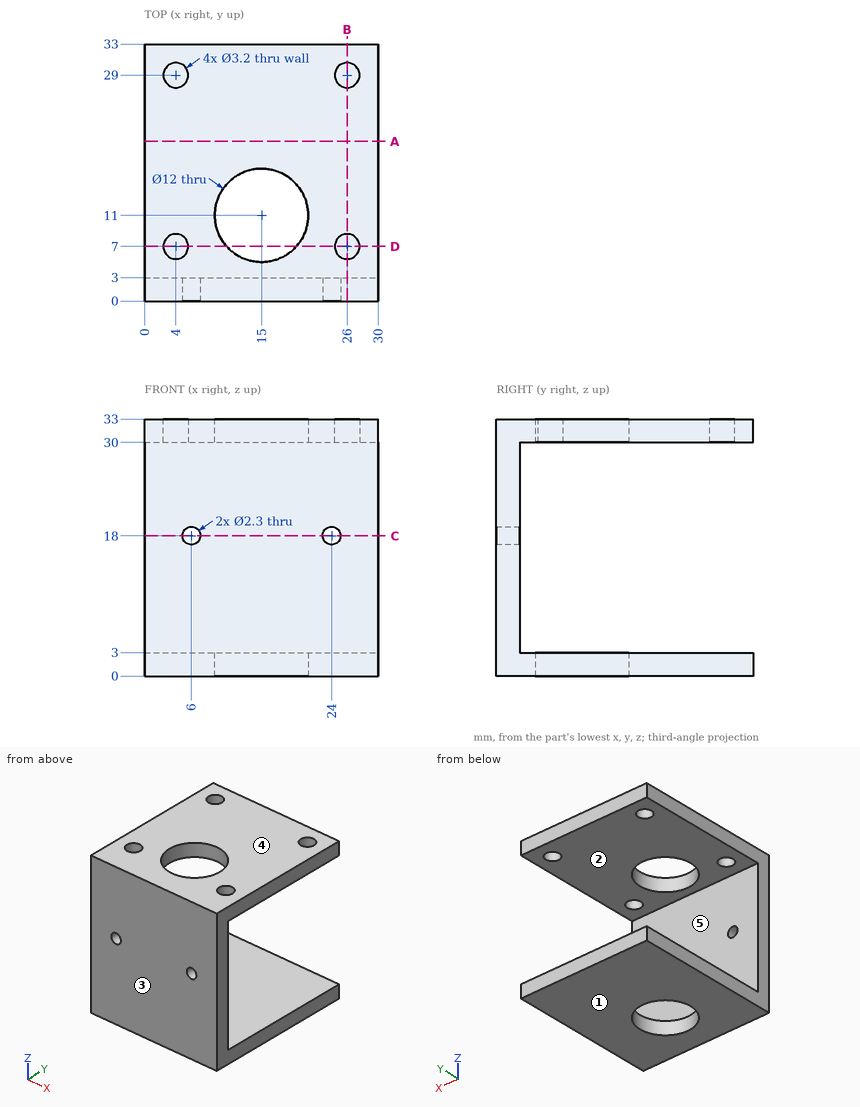
Here's the drawing with two shaded views (mm, measured from the low corner). I have some questions. A direction names the side the tool comes from. Round coordinates to 2 decimals unless told otherwise and drop trailing zeros. Loops run counter-clockwise (first coordinate to the right, second up) from the corner with the lowest first, then second, coordinate; pieces in that order, holes last.
1. Suppose I cut it at D-D, the plane y = 7. Please give me the cut outline in (x, z).
Answers:
outline: (0, 0) - (10.53, 0) - (10.53, 3) - (0, 3) - close; (0, 30) - (2.4, 30) - (2.4, 33) - (0, 33) - close; (5.6, 30) - (10.53, 30) - (10.53, 33) - (5.6, 33) - close; (19.47, 0) - (30, 0) - (30, 3) - (19.47, 3) - close; (19.47, 30) - (24.4, 30) - (24.4, 33) - (19.47, 33) - close; (27.6, 30) - (30, 30) - (30, 33) - (27.6, 33) - close
2. Suppose I cut it at A-A, the plane y = 20.5. Please give me the cut outline in (x, z).
Answers:
outline: (0, 0) - (30, 0) - (30, 3) - (0, 3) - close; (0, 30) - (30, 30) - (30, 33) - (0, 33) - close
3. If I drill on probe 1 along Y at (x, z) = (26, 31.8); probe 2 along X at (y, z) = (1, 18); probe 3 along Z at (x, y) = (24.5, 24), over which ranges is the centre line in solid material (lowest first)?
Answers:
probe 1: y = 0 to 5.4, 8.6 to 27.4, 30.6 to 33
probe 2: x = 0 to 4.85, 7.15 to 22.85, 25.15 to 30
probe 3: z = 0 to 3, 30 to 33
4. Thinking about a two-plate mould opening in Z: for the marked faces 1, 2 and 3, which applies, released by +Z, released by -Z, zero draft, split by the parting line, or undercut?
Answers:
face 1: released by -Z
face 2: undercut
face 3: zero draft
5. Suppose I cut it at B-B, the plane x = 26. Please give me the cut outline in (y, z).
Answers:
outline: (0, 0) - (33, 0) - (33, 3) - (3, 3) - (3, 30) - (5.4, 30) - (5.4, 33) - (0, 33) - close; (8.6, 30) - (27.4, 30) - (27.4, 33) - (8.6, 33) - close; (30.6, 30) - (33, 30) - (33, 33) - (30.6, 33) - close
6. Suppose I cut it at C-C, the plane z = 18. Please give me the cut outline in (x, y).
Answers:
outline: (0, 0) - (4.85, 0) - (4.85, 3) - (0, 3) - close; (7.15, 0) - (22.85, 0) - (22.85, 3) - (7.15, 3) - close; (25.15, 0) - (30, 0) - (30, 3) - (25.15, 3) - close
7. Will these pins go through, and if not, where does the flat tip stop? pin 1 (12 mm diameter, centred on y = 13.5, z = 16.5, fed in from -X); pin 2 (8 mm diameter, centred on x = 21, z = 20.5, fed in from +Y).
Answers:
pin 1: passes through
pin 2: stops at y = 3
8. For the marked faces 4 and 5, which set-ups out of +Z, -Z, +X, -X, +Y, -Y let a thin tool reach every point of the face, with its end or its side?
Answers:
face 4: +Z, +X, -X, +Y, -Y
face 5: +X, -X, +Y
